Design review of the part built by this model. Coordinates are the model's own, in mm. Coordinates: 2 decimals unless noted, no trailing zeros. Write each loop counter-clockwise with the first axis right and the second up, starting at its lowest first coordinate (ties: lowest second). Pieces come first, ordered by that corner, then holes. Notation, with made-up numbers: (49.5, -36) - (95.5, -36) arc R32 cw to (95.5, 0) - close; hole circle Ø3 at (55, 67.5). An arc over 180 degrees is marked (long way). Answer as a JSON object with one key per item and string values.
```python
from build123d import *

# Parameters (mm, degrees)
SKETCH1_R           = 4.7625
BOSS_EXTRUDE1_DEPTH = 107.061
SKETCH2_R           = 5.514901598
SKETCH2_R_2         = 4.4704
CUT_EXTRUDE1_DEPTH  = 0.7366
CUT_EXTRUDE2_START  = 0.7366
SKETCH3_R           = 6.35
SKETCH3_R_2         = 4.4704
CUT_EXTRUDE2_DEPTH  = 0.7366
CHAMFER1_SIZE       = 0.254


with BuildPart() as part:
    # Sketch1 → Boss-Extrude1 (new body)
    with BuildSketch(Plane.XY):
        with Locations(Location((0, 0, 0), (0, 0, 180))):
            Circle(SKETCH1_R)
    extrude(amount=BOSS_EXTRUDE1_DEPTH)

    # Sketch2 → Cut-Extrude1 (cut)
    with BuildSketch(Plane.XY.offset(100.711)):
        Circle(SKETCH2_R)
        Circle(SKETCH2_R_2, mode=Mode.SUBTRACT)
    extrude(amount=CUT_EXTRUDE1_DEPTH, mode=Mode.SUBTRACT)

    # Sketch3 → Cut-Extrude2 (cut)
    with BuildSketch(Plane(origin=(0, 0, 6.35), x_dir=(-1, 0, 0), z_dir=(0, 0, -1)).offset(CUT_EXTRUDE2_START)):
        Circle(SKETCH3_R)
        with Locations(Location((0, 0, 0), (0, 0, 180))):
            Circle(SKETCH3_R_2, mode=Mode.SUBTRACT)
    extrude(amount=-CUT_EXTRUDE2_DEPTH, mode=Mode.SUBTRACT)

    # Chamfer1
    chamfer1_edges = [part.edges().sort_by_distance(p)[0] for p in [
        (4.7625, 0, 0),
        (4.7625, 0, 107.061),
    ]]
    chamfer(chamfer1_edges, length=CHAMFER1_SIZE)


solid = part.part
```
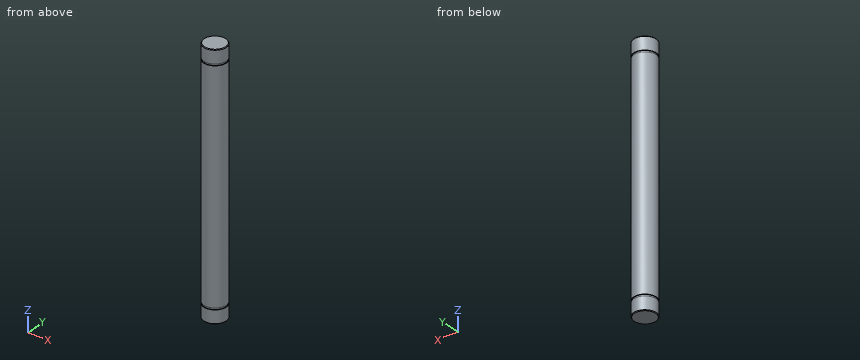
(1) To check wall thickness, follow line 1 (Z direction, x = -2.25, y = 4); line 2 (X direction, y = 0.25, z = 31.5); line 3 (X direction, y = -4, z = 59). State the ranges of each line that lie inside material, in increasing order. Write a range as from..to.
Solved:
{"line 1": "z = 0.08..5.61, 6.35..100.71, 101.45..106.98", "line 2": "x = -4.76..4.76", "line 3": "x = -2.58..2.58"}
(2) For pin 1 (1.5 mm diameter, centred on x = -1, z = 24, fed in from +Y), flat-tipped, find the tip position at first contact; note if it passes through.
Solved:
{"pin 1": "stops at y = 4.76"}
(3) Take a section at A-A, the plane z = 23. Write out the cut boundary in (x, y) (1 decimal).
Solved:
{"outline": "circle Ø9.5 at (0, 0)"}
